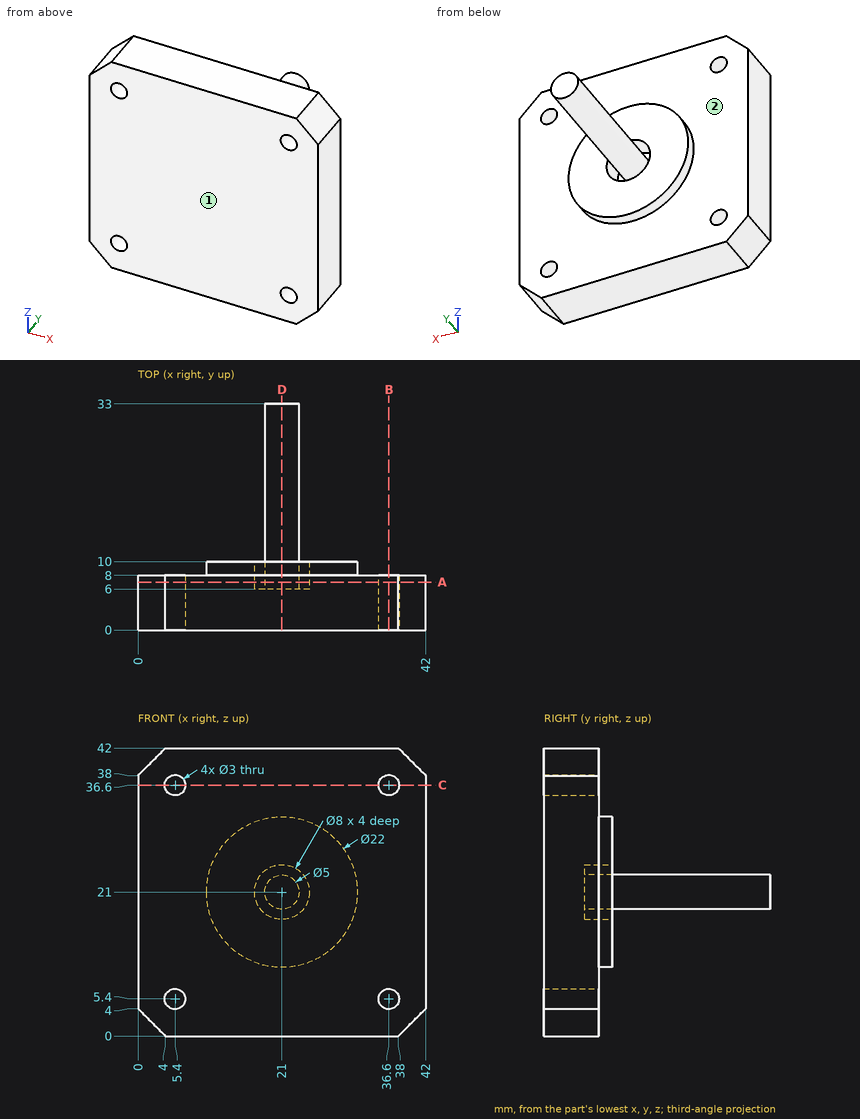
For this review, use the dimensioned drawing (mm, ordinates from the lowest corner) and the shaded views. A direction names the side the tool comes from. Coordinates: 2 decimals unless noted, no trailing zeros. Loops run counter-clockwise (first coordinate to the right, second up) from the corner with the lowest first, then second, coordinate; pieces in that order, holes last. Notation, with made-up numbers: (-4, -7) -> (25, -7) arc R26 ccw to (25, 16) -> close; hole circle Ø5 at (-25.75, 16). An arc over 180 degrees is marked (long way). Use a Markdown table: item, result. Add a question column.
1. Add section C-C on z = 36.6. Write out the cut boundary in (x, y), plus the area to 3 significant figures.
2. To check wall thickness, follow line 1 (Z direction, x = 5.4, y = 2.25); line 2 (Z direction, x = 21, y = 7.55). State the ranges of each line that lie inside material, in increasing order.
3. Clearance check with flat-ended pins moving along their axes: pin 1 Ø6 at (x, z) = (10.5, 12.5) entering from +Y; pin 2 Ø5 at (x, z) = (37.5, 16.5) entering from +Y; pin 3 Ø10 at (y, z) = (20, 23) entering from -X. State where each tip first meets the part, or that it passes through.
4. Machinability: for the marked faces 1 and 2, which of the approach directions +Z, -Z, +X, -X, +Y, -Y give a long, thin tool a straight path to every point of the face, cutting with its end or side? Answer none if there is none.
5. Add section A-A on y = 7. Write out the cut boundary in (x, z).
6. Add section D-D on x = 21. Write out the cut boundary in (y, z), plus the area to 3 significant figures.
7. Add section B-B on x = 36.6. Write out the cut boundary in (y, z).
Returned:
| question | item | result |
|---|---|---|
| 1 | outline | (0, 0) -> (3.9, 0) -> (3.9, 8) -> (0, 8) -> close; (6.9, 0) -> (35.1, 0) -> (35.1, 8) -> (6.9, 8) -> close; (38.1, 0) -> (42, 0) -> (42, 8) -> (38.1, 8) -> close |
| 1 | area | 288 mm² |
| 2 | line 1 | z = 0 to 3.9, 6.9 to 35.1, 38.1 to 42 |
| 2 | line 2 | z = 0 to 17, 18.5 to 23.5, 25 to 42 |
| 3 | pin 1 | stops at y = 10 |
| 3 | pin 2 | stops at y = 8 |
| 3 | pin 3 | stops at x = 18.5 |
| 4 | face 1 | +Z, -Z, +X, -X, -Y |
| 4 | face 2 | +Y |
| 5 | outline | (0, 4) -> (4, 0) -> (38, 0) -> (42, 4) -> (42, 38) -> (38, 42) -> (4, 42) -> (0, 38) -> close; circle Ø5 at (21, 21); hole circle Ø3 at (5.4, 5.4); hole circle Ø3 at (5.4, 36.6); hole circle Ø8 at (21, 21); hole circle Ø3 at (36.6, 5.4); hole circle Ø3 at (36.6, 36.6) |
| 6 | outline | (0, 0) -> (8, 0) -> (8, 10) -> (10, 10) -> (10, 17) -> (6, 17) -> (6, 18.5) -> (33, 18.5) -> (33, 23.5) -> (6, 23.5) -> (6, 25) -> (10, 25) -> (10, 32) -> (8, 32) -> (8, 42) -> (0, 42) -> close |
| 6 | area | 483 mm² |
| 7 | outline | (0, 0) -> (8, 0) -> (8, 3.9) -> (0, 3.9) -> close; (0, 6.9) -> (8, 6.9) -> (8, 35.1) -> (0, 35.1) -> close; (0, 38.1) -> (8, 38.1) -> (8, 42) -> (0, 42) -> close |
